Work out the finished part from the listing and answer in its coordinate system (mm). A direction names the side the tool comes from. Coordinates: 2 decimals unless noted, no trailing zeros. Loops run counter-clockwise (first coordinate to the right, second up) from the corner with the lowest first, then second, coordinate; pieces in that order, holes last. Notation, with made-up numbers: (30, 44) - (38, 44) arc R14 cw to (38, 56) - close; hole circle Ø7 at (25.5, 41). An arc over 180 degrees is marked (long way). Write each question's results on one line, items separated by ' | '. Start each with the question number.
1. A cutting plane is placed at A-A on y = -4.75. Determine the outline of the cut face in (x, z), then the cut area to 3 significant figures.
2. Find the intervals of material crossed by line 1 along X through (y, z) = (-8.5, 14.75); line 2 along Z through (x, y) = (27, 8.75); line 3 along Y through (x, z) = (12, 17.75), in increasing order. Write a range as [from, to].
3. This flat-tipped pin is pushed along its axis until it touches: P1, Ø12, axis at x = 19.5, y = 2.5, coming from the +Z side. Where does it stop, or does it pass through?
4. A cutting plane is placed at D-D on y = 3.25. Determine the outline of the cut face in (x, z), then the cut area to 3 significant figures.
5. A cutting plane is placed at C-C on x = 33. Determine the outline of the cut face in (y, z).
6. A cutting plane is placed at B-B on z = 11.5. Determine the outline of the cut face in (x, y).
7. Which of the six approach directions +Z, -Z, +X, -X, +Y, -Y give full straight-line access (tool end or side, diameter ignored) to faces 1 (the flat face through (38.1, 0, 3)), 2 (the flat face through (12.7, 0, 16))?
from build123d import *

# Parameters (mm, degrees)
F0_W     = 38.1
F0_H     = 25.4
F1_DEPTH = 12.7
F2_W     = 25.4
F2_H     = 19.05
F3_DEPTH = 12.7
F5_DEPTH = 12.7


with BuildPart() as f1:
    # F0 (on Front) → F1 (new body, symmetric)
    with BuildSketch(Plane.XZ):
        with Locations((19.05, 12.7)):
            Rectangle(F0_W, F0_H)
    extrude(amount=F1_DEPTH, both=True)

    # F2 (on Front) → F3 (cut, symmetric)
    with BuildSketch(Plane.XZ):
        with Locations((25.4, 15.875)):
            Rectangle(F2_W, F2_H)
    extrude(amount=F3_DEPTH, both=True, mode=Mode.SUBTRACT)

    # F4 (on Right) → F5 (cut, symmetric)
    with BuildSketch(Plane.YZ):
        with BuildLine():
            ThreePointArc((-12.7, 13.071217), (-9.088983, 21.788983), (-0.371217, 25.4))
            Line((-0.371217, 25.4), (-12.7, 25.4))
            Line((-12.7, 25.4), (-12.7, 13.071217))
        make_face()
        with BuildLine():
            Line((12.7, 25.4), (0.371217, 25.4))
            ThreePointArc((0.371217, 25.4), (9.088983, 21.788983), (12.7, 13.071217))
            Line((12.7, 13.071217), (12.7, 25.4))
        make_face()
    extrude(amount=F5_DEPTH, both=True, mode=Mode.SUBTRACT)


solid = f1.part
Values:
1) outline: (0, 0) - (38.1, 0) - (38.1, 6.35) - (12.7, 6.35) - (12.7, 24.6) - (0, 24.6) - close | area: 474 mm^2
2) line 1: [0, 12.7] | line 2: [0, 6.35] | line 3: [-11.78, 11.78]
3) P1: z = 6.35
4) outline: (0, 0) - (38.1, 0) - (38.1, 6.35) - (12.7, 6.35) - (12.7, 25.06) - (0, 25.06) - close | area: 480 mm^2
5) outline: (-12.7, 0) - (12.7, 0) - (12.7, 6.35) - (-12.7, 6.35) - close
6) outline: (0, -12.7) - (12.7, -12.7) - (12.7, 12.7) - (0, 12.7) - close
7) face 1: +Z, -Z, +X, +Y, -Y | face 2: +Z, +X, +Y, -Y
